The listing builds one solid part. Answer for the finished solid, in the listing's coordinates (mm). A direction names the side the tool comes from. Give positions to 0.01 mm unless a question says otherwise; leave off trailing zeros. Write each loop counter-clockwise with the first axis right and the second up, starting at its lowest first coordinate (ties: lowest second). Pieces come first, ordered by that corner, then holes. Notation, with made-up numbers: (-33, -39.5) - (10, -39.5) arc R20 ccw to (10, -28.5) - close; hole circle Ø7 at (0.5, 1). An arc over 180 degrees is marked (long way). Use a Markdown table: item, result. Add a question column.
from build123d import *

# Parameters (mm, degrees)
EXTRUDE_1_DEPTH          = 3
FILLET_1_R               = 10
FILLET_2_R               = 10
FILLET_3_R               = 10
FILLET_4_R               = 10
SKETCH_2_R               = 1.52
SKETCH_2_R_2             = 4.5
SKETCH_2_W               = 29.255357074
SKETCH_2_H               = 2.887641603
CUT_EXTRUDE_1_DEPTH      = 49
FILLET_5_R               = 20
FILLET_6_R               = 20
PATTERN_CIRCULAR_2_COUNT = 4
SKETCH_3_R               = 10
CUT_EXTRUDE_2_DEPTH      = 49
FILLET_7_R               = 20
FILLET_8_R               = 20
FILLET_9_R               = 20
FILLET_10_R              = 20
FILLET_11_R              = 20
FILLET_12_R              = 20


with BuildPart() as part:
    # 草图1 → 凸台-拉伸1 (new body)
    with BuildSketch(Plane(origin=(0, 0, 0), x_dir=(1, 0, 0), z_dir=(0, 1, 0))):
        with BuildLine():
            Line((60.104076401, -60.104076401), (36.583704196, -60.104076401))
            ThreePointArc((36.583704196, -60.104076401), (0, -37.75481759), (-36.583704196, -60.104076401))
            Line((-36.583704196, -60.104076401), (-60.104076401, -60.104076401))
            Line((-60.104076401, -60.104076401), (-60.104076401, -36.583704196))
            ThreePointArc((-60.104076401, -36.583704196), (-37.75481759, 0), (-60.104076401, 36.583704196))
            Line((-60.104076401, 36.583704196), (-60.104076401, 60.104076401))
            Line((-60.104076401, 60.104076401), (-36.583704196, 60.104076401))
            ThreePointArc((-36.583704196, 60.104076401), (0, 37.75481759), (36.583704196, 60.104076401))
            Line((36.583704196, 60.104076401), (60.104076401, 60.104076401))
            Line((60.104076401, 60.104076401), (60.104076401, 36.583704196))
            ThreePointArc((60.104076401, 36.583704196), (37.75481759, 0), (60.104076401, -36.583704196))
            Line((60.104076401, -36.583704196), (60.104076401, -60.104076401))
        make_face()
    extrude(amount=EXTRUDE_1_DEPTH)

    # 圆角1
    fillet_1_edges = [part.edges().sort_by_distance(p)[0] for p in [
        (60.104076401, 1.5, 60.104076401),
    ]]
    fillet(fillet_1_edges, radius=FILLET_1_R)

    # 圆角2
    fillet_2_edges = [part.edges().sort_by_distance(p)[0] for p in [
        (60.104076401, 1.5, -60.104076401),
    ]]
    fillet(fillet_2_edges, radius=FILLET_2_R)

    # 圆角3
    fillet_3_edges = [part.edges().sort_by_distance(p)[0] for p in [
        (-60.104076401, 1.5, -60.104076401),
    ]]
    fillet(fillet_3_edges, radius=FILLET_3_R)

    # 圆角4
    fillet_4_edges = [part.edges().sort_by_distance(p)[0] for p in [
        (-60.104076401, 1.5, 60.104076401),
    ]]
    fillet(fillet_4_edges, radius=FILLET_4_R)

    # 草图2 → 切除-拉伸1 (cut)
    with BuildSketch(Plane(origin=(0, 3, 0), x_dir=(1, 0, 0), z_dir=(0, 1, 0))):
        with Locations(Location((-27.792783788, 34.8638516, 0), (0, 0, 270))):
            Circle(SKETCH_2_R)
        with Locations(Location((-34.8638516, 27.792783788, 0), (0, 0, 270))):
            Circle(SKETCH_2_R)
        with Locations(Location((-40.073266213, 40.073266213, 0), (0, 0, 270))):
            Circle(SKETCH_2_R_2)
        with Locations(Location((-46.88466688, 53.955734692, 0), (0, 0, 270))):
            Circle(SKETCH_2_R)
        with Locations(Location((-53.955734692, 46.88466688, 0), (0, 0, 270))):
            Circle(SKETCH_2_R)
        with Locations((0, 24.84759336)):
            Rectangle(SKETCH_2_W, SKETCH_2_H)
    cut_extrude_1 = extrude(amount=-CUT_EXTRUDE_1_DEPTH, mode=Mode.SUBTRACT)

    # 圆角5
    fillet_5_edges = [part.edges().sort_by_distance(p)[0] for p in [
        (-36.583704196, 1.5, -60.104076401),
    ]]
    fillet(fillet_5_edges, radius=FILLET_5_R)

    # 圆角6
    fillet_6_edges = [part.edges().sort_by_distance(p)[0] for p in [
        (-60.104076401, 1.5, -36.583704196),
    ]]
    fillet(fillet_6_edges, radius=FILLET_6_R)

    # 阵列(圆周)2: 切除-拉伸1 ×4 about axis
    pattern_circular_2_axis = Axis((0, 0, 0), (0, 1, 0))
    for i in range(1, PATTERN_CIRCULAR_2_COUNT):
        add(cut_extrude_1.rotate(pattern_circular_2_axis, i * 360 / PATTERN_CIRCULAR_2_COUNT), mode=Mode.SUBTRACT)

    # 草图3 → 切除-拉伸2 (cut)
    with BuildSketch(Plane(origin=(0, 3, 0), x_dir=(1, 0, 0), z_dir=(0, 1, 0))):
        with Locations(Location((0, 0, 0), (0, 0, 270))):
            Circle(SKETCH_3_R)
    extrude(amount=-CUT_EXTRUDE_2_DEPTH, mode=Mode.SUBTRACT)

    # 圆角7
    fillet_7_edges = [part.edges().sort_by_distance(p)[0] for p in [
        (60.104076401, 1.5, 36.583704196),
    ]]
    fillet(fillet_7_edges, radius=FILLET_7_R)

    # 圆角8
    fillet_8_edges = [part.edges().sort_by_distance(p)[0] for p in [
        (36.583704196, 1.5, 60.104076401),
    ]]
    fillet(fillet_8_edges, radius=FILLET_8_R)

    # 圆角9
    fillet_9_edges = [part.edges().sort_by_distance(p)[0] for p in [
        (-60.104076401, 1.5, 36.583704196),
    ]]
    fillet(fillet_9_edges, radius=FILLET_9_R)

    # 圆角10
    fillet_10_edges = [part.edges().sort_by_distance(p)[0] for p in [
        (-36.583704196, 1.5, 60.104076401),
    ]]
    fillet(fillet_10_edges, radius=FILLET_10_R)

    # 圆角11
    fillet_11_edges = [part.edges().sort_by_distance(p)[0] for p in [
        (36.583704196, 1.5, -60.104076401),
    ]]
    fillet(fillet_11_edges, radius=FILLET_11_R)

    # 圆角12
    fillet_12_edges = [part.edges().sort_by_distance(p)[0] for p in [
        (60.104076401, 1.5, -36.583704196),
    ]]
    fillet(fillet_12_edges, radius=FILLET_12_R)


solid = part.part
1. Given P1, Ø12, axis at x = 0, z = 0, coming from the +Y side (3 decimals); P2, Ø1, axis at y = 1, z = 4, coming from the -X side; P3, Ø1, axis at y = 0.5, z = 22.5, coming from the -X side; P4, Ø0.9, axis at x = -6.5, y = 2, coming from the +Z side, each flat-ended and moving along its own axis, determine where each tip first touches the part or whether it passes through.
2. The part is cut by section C-C (y = 0.65). Count the separate pieces of the cut face and the enclosed holes in it, and give its area (3 significant figures).
3. The part is cut by section B-B (z = 0). Give the vertices of the cut face in (x, y).
4. The part is cut by section A-A (x = 0). Give the vertices of the cut face in (y, z), and give its area (3 significant figures).
5. Which of the six approach directions +Z, -Z, +X, -X, +Y, -Y give full straight-line access (tool end or side, diameter ignored) to faces 1 (the flat face through (-23.404, 2, 0)), 2 (the cylindrical face through (38.808, 1.521, 58.236)), 3 (the cylindrical face through (57.1, 1.52, 57.25))?
6. Consider L1, parallel to Z at x = -47.5, y = 2.5; L2, parallel to X at y = 0.6, z = -0.5; L3, parallel to Z at x = -6, y = 2.85. Determine where each line is inside the solid, lowest interval first. Write a range as [from, to].
7. The part is cut by section D-D (z = 22). Give the vertices of the cut face in (x, y).
8. For a pull along X with two mould halves and no side action, classify faces 4 (the flat face through (-13, 3, -1)), 5 (the cylindrical face through (28.72, 1.52, 36.07)), 6 (the cylindrical face through (58.236, 1.521, -38.808)), 7 (the flat face through (0, 2, -23.404)) as released by +X, released by -X, zero draft, split by the parting line, or undercut.
Check values:
| question | item | result |
|---|---|---|
| 1 | P1 | passes through |
| 1 | P2 | stops at x = -38 |
| 1 | P3 | stops at x = -44.79 |
| 1 | P4 | stops at z = 38.35 |
| 2 | separate pieces | 1 |
| 2 | enclosed holes | 25 |
| 2 | area | 8,550 mm2 |
| 3 | outline | (-37.75, 0) - (-26.29, 0) - (-26.29, 3) - (-37.75, 3) - close; (-23.4, 0) - (-10, 0) - (-10, 3) - (-23.4, 3) - close; (10, 0) - (23.4, 0) - (23.4, 3) - (10, 3) - close; (26.29, 0) - (37.75, 0) - (37.75, 3) - (26.29, 3) - close |
| 4 | outline | (0, -37.75) - (3, -37.75) - (3, -26.29) - (0, -26.29) - close; (0, -23.4) - (3, -23.4) - (3, -10) - (0, -10) - close; (0, 10) - (3, 10) - (3, 23.4) - (0, 23.4) - close; (0, 26.29) - (3, 26.29) - (3, 37.75) - (0, 37.75) - close |
| 4 | area | 149 mm2 |
| 5 | face 1 | +Y, -Y |
| 5 | face 2 | +Z, +Y, -Y |
| 5 | face 3 | +Z, +X, +Y, -Y |
| 6 | L1 | z = [-60.1, -55.35], [-52.57, -26.58], [26.58, 52.57], [55.35, 60.1] |
| 6 | L2 | x = [-37.76, -26.29], [-23.4, -9.99], [9.99, 23.4], [26.29, 37.76] |
| 6 | L3 | z = [-38.19, -26.29], [-23.4, -8], [8, 23.4], [26.29, 38.19] |
| 7 | outline | (-44.14, 0) - (44.14, 0) - (44.14, 3) - (-44.14, 3) - close |
| 8 | face 4 | zero draft |
| 8 | face 5 | undercut |
| 8 | face 6 | released by +X |
| 8 | face 7 | undercut |
